Source: CAD feature listing. Evaluate the final solid. Frame: model axes, mm. Coordinates: 2 decimals unless noted, no trailing zeros. Write each loop counter-clockwise with the first axis right and the second up, starting at its lowest first coordinate (ties: lowest second). Pieces come first, ordered by that corner, then holes. Notation, with made-up numbers: M 35,-15 L 75,-15 A19 cw 75,13 Z; hole C 13.25,66 d8. An arc over 180 degrees is marked long. One line per item, written item: value. Start each with the question number.
Item 1: Pin query (flat end, axial travel): P1, Ø4, axis at x = -88.5, z = 30, coming from the +Y side. Return the tip coordinate at first contact, or that it passes through.
Item 2: Ray query, L1, parallel to X at y = 0.4, z = 30; L2, parallel to X at y = 0.55, z = 0. Return the intervals inside material, ascending. Write a range as from..to.
Item 3: Mould query, pull axis Z, two halves, no side actions, for faces 1 (the flat face through (-1, 0, -1)), 2 (the cylindrical face through (90.88, 0.51, -0.31)). Classes: released by +Z, released by -Z, zero draft, split by the parting line, or undercut.
Item 4: Cut plane B-B, the plane z = 30. Output: boundary loops of the cut face in (x, y), then the cut area to 3 significant figures.
Item 5: Cut plane A-A, the plane x = -88.5. Output: boundary loops of the cut face in (y, z).
```python
from build123d import *

# Parameters (mm, degrees)
SKETCH1_W           = 189
SKETCH1_H           = 132
BOSS_EXTRUDE1_DEPTH = 1
SKETCH3_R           = 2.4
CUT_EXTRUDE1_DEPTH  = 116.270334432
FILLET1_R           = 3


with BuildPart() as part:
    # Sketch1 → Boss-Extrude1 (new body)
    with BuildSketch(Plane(origin=(0, 0, 0), x_dir=(1, 0, 0), z_dir=(0, 1, 0))):
        Rectangle(SKETCH1_W, SKETCH1_H)
    extrude(amount=BOSS_EXTRUDE1_DEPTH)

    # Sketch3 → Cut-Extrude1 (cut, through all)
    with BuildSketch(Plane(origin=(0, 1, 0), x_dir=(1, 0, 0), z_dir=(0, 1, 0))):
        with Locations(Location((88.5, 0, 0), (0, 0, 270))):
            Circle(SKETCH3_R)
        with Locations(Location((-88.5, -30, 0), (0, 0, 270))):
            Circle(SKETCH3_R)
        with Locations(Location((-88.5, 30, 0), (0, 0, 270))):
            Circle(SKETCH3_R)
    extrude(amount=-CUT_EXTRUDE1_DEPTH, mode=Mode.SUBTRACT)

    # Fillet1
    fillet1_edges = [part.edges().sort_by_distance(p)[0] for p in [
        (94.5, 0.5, 66),
        (-94.5, 0.5, 66),
        (-94.5, 0.5, -66),
        (94.5, 0.5, -66),
    ]]
    fillet(fillet1_edges, radius=FILLET1_R)


solid = part.part
```
From the geometry:
1. P1: passes through
2. L1: x = -94.5..-90.9, -86.1..94.5
2. L2: x = -94.5..86.1, 90.9..94.5
3. face 1: zero draft
3. face 2: undercut
4. outline: M -94.5,0 L -90.9,0 L -90.9,1 L -94.5,1 Z; M -86.1,0 L 94.5,0 L 94.5,1 L -86.1,1 Z
4. area: 184 mm²
5. outline: M 0,-66 L 1,-66 L 1,-32.4 L 0,-32.4 Z; M 0,-27.6 L 1,-27.6 L 1,27.6 L 0,27.6 Z; M 0,32.4 L 1,32.4 L 1,66 L 0,66 Z
